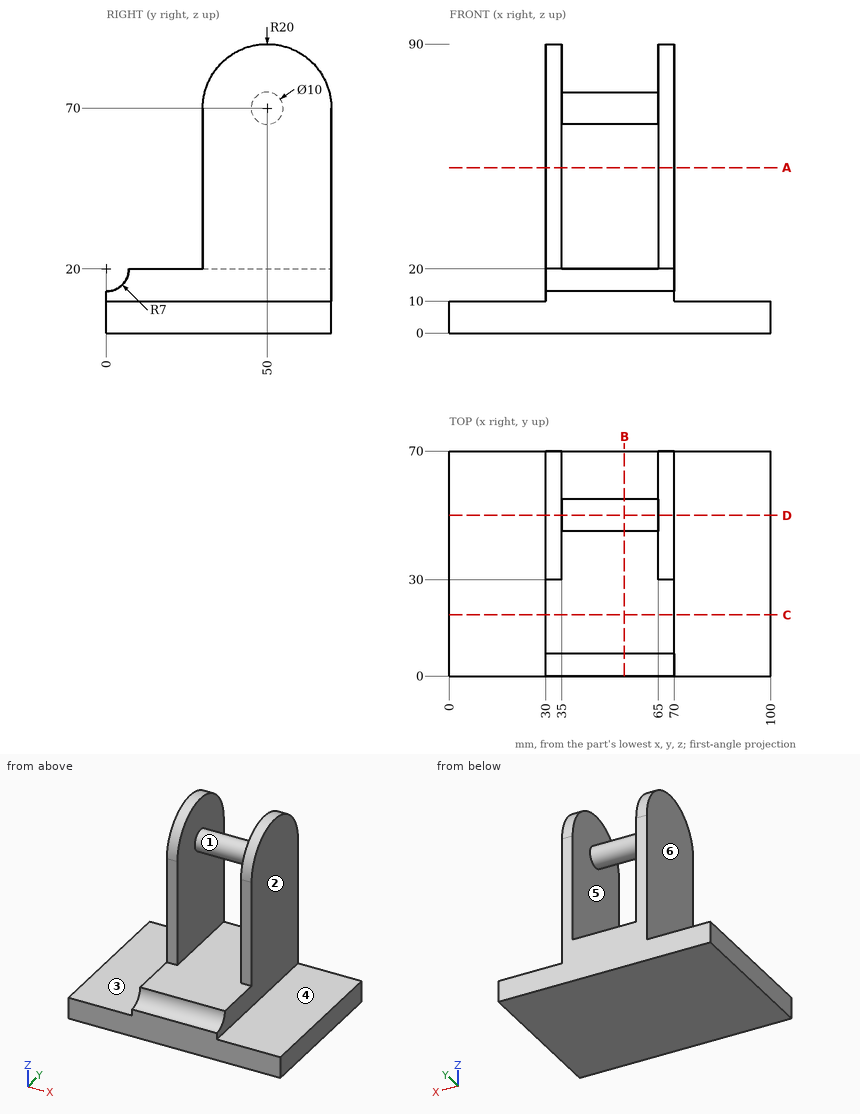
Check sheet for the drawn part. Datum: minimum x, y, z corner. Units: mm. A direction names the side the tool comes from. Give positions to 0.01 mm unless a question says otherwise; leave off trailing zeros. Order: outer loops, then holes, each group sorted by start corner. A loop starts at its lowest first (then second) coordinate and runs counter-clockwise, first axis right, second up. Notation, with made-up numbers: (10.25, 87) - (22.25, 87) arc R8 ccw to (22.25, 96) - close; hole circle Ø5 at (56, 44). An arc over 180 degrees is marked (long way). Answer in a Markdown table with one row per item. Add a question column.
Q1. Cross-section at B-B, the plane x = 54.5. Enter the section's corners in (y, z).
Q2. Cross-section at C-C, the plane y = 19. Enter the section's corners in (x, z), then the cut area to 3 significant figures.
Q3. Cross-section at A-A, the plane z = 51.5. Enter the section's corners in (x, y), then the cut area to 3 significant figures.
Q4. Tool access check on the marked faces 1, 2 and 3. Record the directions out of +Z, -Z, +X, -X, +Y, -Y that give a thin tool (end or side, any length) a straight path to the whole face; none if there is none.
Q5. Mould release check, pull along Z, two halves, no side actions. Record for the marked faces 4, 5 and 6: pulls with the +Z half, pulls with the -Z half, needs draft (parallel to the pull), parting line crosses it, or undercut.
Q6. Gauge pin test, flat ends, axial feed: pin 1 (3 mm diameter, centred on y = 38.5, z = 55, fed in from +X); pin 2 (6 mm diameter, centred on x = 68.5, z = 51.5, fed in from -Y); pin 3 (15 mm diameter, centred on x = 8.5, y = 23.5, fed in from +Z). Record the tip position at first contact, or that the pin passes through.
Q7. Cross-section at D-D, the plane y = 50. Enter the section's corners in (x, z).
Q8. Material ranges on probe 1 along X at (y, z) = (40, 50.5); probe 2 along Z at (x, y) = (25.5, 26); probe 3 along Z at (x, y) = (57, 27.5), recorded low to high. Write a range as from..to.
Check values:
| question | item | result |
|---|---|---|
| 1 | outline | (0, 0) - (70, 0) - (70, 20) - (7, 20) arc R7 cw to (0, 13) - close; circle Ø10 at (50, 70) |
| 2 | outline | (0, 0) - (100, 0) - (100, 10) - (70, 10) - (70, 20) - (30, 20) - (30, 10) - (0, 10) - close |
| 2 | area | 1,400 mm^2 |
| 3 | outline | (30, 30) - (35, 30) - (35, 70) - (30, 70) - close; (65, 30) - (70, 30) - (70, 70) - (65, 70) - close |
| 3 | area | 400 mm^2 |
| 4 | face 1 | none |
| 4 | face 2 | +Z, +X, +Y, -Y |
| 4 | face 3 | +Z, -X, +Y, -Y |
| 5 | face 4 | pulls with the +Z half |
| 5 | face 5 | undercut |
| 5 | face 6 | needs draft |
| 6 | pin 1 | stops at x = 70 |
| 6 | pin 2 | stops at y = 30 |
| 6 | pin 3 | stops at z = 10 |
| 7 | outline | (0, 0) - (100, 0) - (100, 10) - (70, 10) - (70, 90) - (65, 90) - (65, 75) - (35, 75) - (35, 90) - (30, 90) - (30, 10) - (0, 10) - close; hole (35, 20) - (65, 20) - (65, 65) - (35, 65) - close |
| 8 | probe 1 | x = 30..35, 65..70 |
| 8 | probe 2 | z = 0..10 |
| 8 | probe 3 | z = 0..20 |
